The listing builds one solid part. Answer for the finished solid, in the listing's coordinates (mm). A direction names the side the tool comes from. Give positions to 0.01 mm unless a question says otherwise; leave off trailing zeros. Loops run counter-clockwise (first coordinate to the right, second up) from the corner with the lowest first, then second, coordinate; pieces in that order, holes last. Notation, with made-up numbers: (58.5, 0.25) - (77.5, 0.25) arc R36 cw to (77.5, 37.25) - close; hole circle Ø10 at (40, 32). An arc over 180 degrees is marked (long way). One line per item, written item: value. Start each with the question number.
from build123d import *

# Parameters (mm, degrees)
F0_R     = 1
F1_DEPTH = 1


# Not quite as in the source:
# - a feature names something its author has since deleted; it is built from what else it names


with BuildPart() as f1:
    # F0 (on Right) → F1 (new body)
    with BuildSketch(Plane.YZ):
        Polygon((8.384144865, 0), (0, 0), (0, -11.5), (11.5, -11.5), (11.5, 0), (10.384144865, 0), (10.384144865, 10), (8.384144865, 10), align=None)
        with Locations((3.25, -8.25)):
            Circle(F0_R, mode=Mode.SUBTRACT)
        with Locations((3.25, -5.75)):
            Circle(F0_R, mode=Mode.SUBTRACT)
        with Locations((3.25, -3.25)):
            Circle(F0_R, mode=Mode.SUBTRACT)
        with Locations((5.75, -8.25)):
            Circle(F0_R, mode=Mode.SUBTRACT)
        with Locations((8.25, -8.25)):
            Circle(F0_R, mode=Mode.SUBTRACT)
        with Locations((5.75, -5.75)):
            Circle(F0_R, mode=Mode.SUBTRACT)
        with Locations((8.25, -5.75)):
            Circle(F0_R, mode=Mode.SUBTRACT)
        with Locations((5.75, -3.25)):
            Circle(F0_R, mode=Mode.SUBTRACT)
        with Locations((8.25, -3.25)):
            Circle(F0_R, mode=Mode.SUBTRACT)
    extrude(amount=F1_DEPTH)


solid = f1.part
1. Flat-ended cylindrical pins translate along their axes: pin 1 (2.5 mm diameter, centred on y = 8.25, z = -5.75, fed in from -X); pin 2 (1.6 mm diameter, centred on y = 3.25, z = -8.25, fed in from +X); pin 3 (0.5 mm diameter, centred on x = 0.5, z = 5.5, fed in from +Y); pin 4 (0.5 mm diameter, centred on x = 0.5, y = 6, fed in from +Z). Find the tip coordinate at first contact, or state that the pin passes through.
2. For faces 1 (the flat face through (0.5, 10.9, 0)), 2 (the flat face through (0.5, 8.384, 5.1)), 3 (the flat face through (0.5, 11.5, -5.8)), determine the directions among +Z, -Z, +X, -X, +Y, -Y from which every point of the face is accessible in a straight line to the end or side of a thin tool.
3. A cutting plane is placed at C-C (x = 0.3). Give the number of separate pieces and of enclosed holes in the cut face, plus the area to 3 significant figures.
4. A cutting plane is placed at B-B (y = 3.25). Determine the outline of the cut face in (x, z).
5. A cutting plane is placed at A-A (z = -8.25). Determine the outline of the cut face in (x, y).
6. A cutting plane is placed at D-D (z = 2.75). Determine the outline of the cut face in (x, y).
7. Find the intervals of material crossed by L1, parallel to Z at x = 0.65, y = 5.75; L2, parallel to Y at x = 0.65, z = -3.75; L3, parallel to Y at x = 0.35, z = 5.5, in increasing order. Write a range as [from, to].
8. Determine the mould class of faces 4 (the cylindrical face through (0.49, 4.96, -3.86)), 5 (the cylindrical face through (0.49, 3.12, -4.76)), 6 (the flat face through (0.5, 10.384, 4.9)), 7 (the flat face through (0.5, 5.7, -11.5)) for opening direction Z: released by +Z, released by -Z, zero draft, split by the parting line, or undercut.
Results below:
1. pin 1: stops at x = 0
1. pin 2: passes through
1. pin 3: stops at y = 10.38
1. pin 4: stops at z = 0
2. face 1: +Z, +X, -X, +Y
2. face 2: +Z, +X, -X, -Y
2. face 3: +Z, -Z, +X, -X, +Y
3. separate pieces: 1
3. enclosed holes: 9
3. area: 124 mm^2
4. outline: (0, -11.5) - (1, -11.5) - (1, -9.25) - (0, -9.25) - close; (0, -7.25) - (1, -7.25) - (1, -6.75) - (0, -6.75) - close; (0, -4.75) - (1, -4.75) - (1, -4.25) - (0, -4.25) - close; (0, -2.25) - (1, -2.25) - (1, 0) - (0, 0) - close
5. outline: (0, 0) - (1, 0) - (1, 2.25) - (0, 2.25) - close; (0, 4.25) - (1, 4.25) - (1, 4.75) - (0, 4.75) - close; (0, 6.75) - (1, 6.75) - (1, 7.25) - (0, 7.25) - close; (0, 9.25) - (1, 9.25) - (1, 11.5) - (0, 11.5) - close
6. outline: (0, 8.38) - (1, 8.38) - (1, 10.38) - (0, 10.38) - close
7. L1: z = [-11.5, -9.25], [-7.25, -6.75], [-4.75, -4.25], [-2.25, 0]
7. L2: y = [0, 2.38], [4.12, 4.88], [6.62, 7.38], [9.12, 11.5]
7. L3: y = [8.38, 10.38]
8. face 4: undercut
8. face 5: undercut
8. face 6: zero draft
8. face 7: released by -Z
